```python
from build123d import *

# Parameters (mm, degrees)
SKETCH1_W      = 50.8
SKETCH1_H      = 60.325
EXTRUDE2_DEPTH = 2.286


with BuildPart() as part:
    # Sketch1 → Extrude2 (new body)
    with BuildSketch(Plane.XY):
        with Locations((25.4, 30.1625)):
            Rectangle(SKETCH1_W, SKETCH1_H)
        with BuildLine():
            Line((5.886865084, 15.264808366), (13.163134916, 15.264808366))
            ThreePointArc((13.163134916, 15.264808366), (14.95918614, 14.52085959), (15.703134916, 12.724808366))
            Line((15.703134916, 12.724808366), (15.703134916, 6.325191634))
            ThreePointArc((15.703134916, 6.325191634), (14.95918614, 4.52914041), (13.163134916, 3.785191634))
            Line((13.163134916, 3.785191634), (5.886865084, 3.785191634))
            ThreePointArc((5.886865084, 3.785191634), (4.09081386, 4.52914041), (3.346865084, 6.325191634))
            Line((3.346865084, 6.325191634), (3.346865084, 12.724808366))
            ThreePointArc((3.346865084, 12.724808366), (4.09081386, 14.52085959), (5.886865084, 15.264808366))
        make_face(mode=Mode.SUBTRACT)
    extrude(amount=-EXTRUDE2_DEPTH)


solid = part.part
```
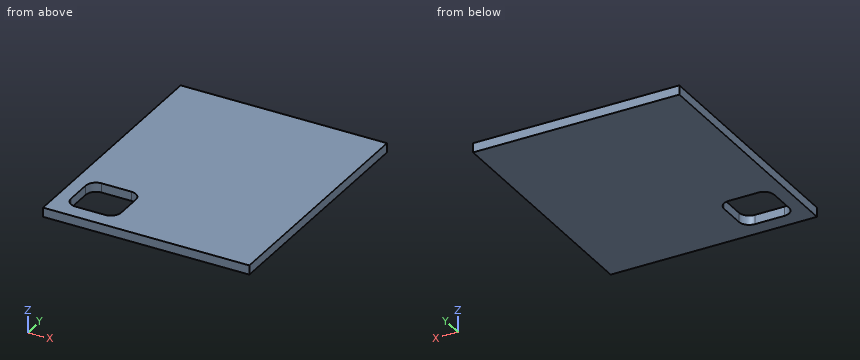
The model under review builds one solid part; all positions refer to its coordinate system, in mm. Round coordinates to 2 decimals unless told otherwise and drop trailing zeros. Loops run counter-clockwise (first coordinate to the right, second up) from the corner with the lowest first, then second, coordinate; pieces in that order, holes last. Notation, with made-up numbers: (35, 31.25) -> (47, 31.25) arc R20 cw to (47, 54.25) -> close; hole circle Ø7 at (53.5, 58). An arc over 180 degrees is marked (long way). Answer as a JSON object with one key per item and string values. Group by question number.
1) For pin 1 Ø1.1 at (x, z) = (10.5, -1) entering from -Y, flat-tipped, find the tip position at first contact; note if it passes through.
2) We need section A-A on x = 12.5. Write out the cut boundary in (y, z) (3 decimals).
3) We need section B-B on z = -0.9. Write out the cut boundary in (x, y) (3 decimals), then the cut area to 3 significant figures.
4) For line 1 (X direction, y = 13, z = -1); line 2 (Y direction, x = 7, z = -0.5) (3 decimals); line 3 (Y direction, x = 5.5, z = -0.35) (3 decimals), list the stretches that pass through material, from the lowest coordinate up. Write a range as [from, to].
5) We need section C-C on x = 5. Write out the cut boundary in (y, z) (3 decimals), then the cut area to 3 significant figures.
Result set:
{
 "1": {"pin 1": "y = 0"},
 "2": {"outline": "(0, -2.286) -> (3.785, -2.286) -> (3.785, 0) -> (0, 0) -> close; (15.265, -2.286) -> (60.325, -2.286) -> (60.325, 0) -> (15.265, 0) -> close"},
 "3": {"outline": "(0, 0) -> (50.8, 0) -> (50.8, 60.325) -> (0, 60.325) -> close; hole (3.347, 6.325) arc R2.54 ccw to (5.887, 3.785) -> (13.163, 3.785) arc R2.54 ccw to (15.703, 6.325) -> (15.703, 12.725) arc R2.54 ccw to (13.163, 15.265) -> (5.887, 15.265) arc R2.54 ccw to (3.347, 12.725) -> close", "area": "2,930 mm²"},
 "4": {"line 1": "[0, 3.36], [15.69, 50.8]", "line 2": "[0, 3.785], [15.265, 60.325]", "line 3": "[0, 3.815], [15.235, 60.325]"},
 "5": {"outline": "(0, -2.286) -> (3.945, -2.286) -> (3.945, 0) -> (0, 0) -> close; (15.105, -2.286) -> (60.325, -2.286) -> (60.325, 0) -> (15.105, 0) -> close", "area": "112 mm²"}
}
